```python
from build123d import *

# Parameters (mm, degrees)
SKETCH1_R           = 69.948062861
BOSS_EXTRUDE1_DEPTH = 25.4
BOSS_EXTRUDE2_DEPTH = 25.4


with BuildPart() as part:
    # Sketch1 → Boss-Extrude1 (new body)
    with BuildSketch(Plane(origin=(0, 0, 0), x_dir=(1, 0, 0), z_dir=(0, 1, 0))):
        with BuildLine():
            ThreePointArc((63.74187476, -40.530752622), (65.16096079, -41.118557302), (66.58004682, -40.530752622))
            ThreePointArc((66.58004682, -40.530752622), (14.23733744, 76.635127489), (-76.694663108, -13.913058378))
            Line((-76.694663108, -13.913058378), (-73.000086536, -13.913058378))
            Line((-73.000086536, -13.913058378), (-75.252390768, -15.474368763))
            Line((-75.252390768, -15.474368763), (-70.740426062, -15.474368763))
            Line((-70.740426062, -15.474368763), (-70.080138544, -17.015039639))
            Line((-70.080138544, -17.015039639), (-72.166015782, -17.521478191))
            Line((-72.166015782, -17.521478191), (-71.123077163, -18.775806353))
            Line((-71.123077163, -18.775806353), (-70.740426062, -20.351838073))
            Line((-70.740426062, -20.351838073), (-71.268418719, -21.218426764))
            Line((-71.268418719, -21.218426764), (-72.996408415, -24.608346096))
            Line((-72.996408415, -24.608346096), (-73.573552306, -25.740569997))
            ThreePointArc((-73.573552306, -25.740569997), (-15.15436006, -76.459073457), (58.193519931, -51.857099617))
            Line((58.193519931, -51.857099617), (58.193519931, -44.265552602))
            Line((58.193519931, -44.265552602), (60.00707478, -44.265552602))
            Line((60.00707478, -44.265552602), (63.74187476, -40.530752622))
        make_face()
        with Locations(Location((0, 0, 0), (0, 0, 90))):
            Circle(SKETCH1_R, mode=Mode.SUBTRACT)
    extrude(amount=BOSS_EXTRUDE1_DEPTH)

    # Sketch2 → Boss-Extrude2 (add)
    with BuildSketch(Plane.XZ):
        with BuildLine():
            Line((16.91938422, -42.867763876), (15.301396265, -46.734397981))
            Line((15.301396265, -46.734397981), (23.266647688, -65.965101405))
            ThreePointArc((23.266647688, -65.965101405), (27.508582432, -64.311813771), (31.633980927, -62.386078164))
            Line((31.633980927, -62.386078164), (22.646440609, -42.05853708))
            Line((22.646440609, -42.05853708), (22.122487474, -44.43690451))
            Line((22.122487474, -44.43690451), (19.98105683, -41.085378254))
            Line((19.98105683, -41.085378254), (19.154678805, -40.246982073))
            Line((19.154678805, -40.246982073), (19.154678805, -42.867763876))
            Line((19.154678805, -42.867763876), (17.562717892, -44.43690451))
            Line((17.562717892, -44.43690451), (16.91938422, -42.867763876))
        make_face()
        with BuildLine():
            Line((7.295677294, -27.358886688), (14.085059503, -43.790609078))
            Line((14.085059503, -43.790609078), (14.802816622, -40.246982073))
            Line((14.802816622, -40.246982073), (16.254758128, -40.541070969))
            Line((16.254758128, -40.541070969), (16.507439862, -39.293560089))
            Line((16.507439862, -39.293560089), (17.562717892, -39.293560089))
            Line((17.562717892, -39.293560089), (17.562717892, -38.21621684))
            Line((17.562717892, -38.21621684), (19.98105683, -38.7060483))
            Line((19.98105683, -38.7060483), (20.801456059, -37.88564907))
            Line((20.801456059, -37.88564907), (12.224600097, -18.486972039))
            ThreePointArc((12.224600097, -18.486972039), (17.735408563, -13.291511043), (21.175132345, -6.543909602))
            Line((21.175132345, -6.543909602), (68.757486976, -12.850660789))
            ThreePointArc((68.757486976, -12.850660789), (69.448887589, -8.341673136), (69.844918996, -3.797207976))
            Line((69.844918996, -3.797207976), (22.122487474, 1.343328216))
            ThreePointArc((22.122487474, 1.343328216), (20.3784905, 8.713558841), (16.254758128, 15.066247738))
            Line((16.254758128, 15.066247738), (22.122487474, 22.699365292))
            Line((22.122487474, 22.699365292), (22.122487474, 30.322912753))
            Line((22.122487474, 30.322912753), (17.562717892, 30.322912753))
            Line((17.562717892, 30.322912753), (9.897887376, 19.830300255))
            ThreePointArc((9.897887376, 19.830300255), (2.643081937, 22.005069884), (-4.920374217, 21.610157341))
            Line((-4.920374217, 21.610157341), (-16.826086698, 50.424467144))
            Line((-16.826086698, 50.424467144), (-17.435403285, 50.17270515))
            Line((-17.435403285, 50.17270515), (-19.742011126, 52.479312991))
            Line((-19.742011126, 52.479312991), (-20.850502701, 50.169534038))
            Line((-20.850502701, 50.169534038), (-23.249744789, 47.77029195))
            Line((-23.249744789, 47.77029195), (-24.874918704, 47.098790412))
            Line((-24.874918704, 47.098790412), (-12.224600097, 18.486972039))
            ThreePointArc((-12.224600097, 18.486972039), (-17.735408563, 13.291511043), (-21.175132345, 6.543909602))
            Line((-21.175132345, 6.543909602), (-68.757486976, 12.850660789))
            ThreePointArc((-68.757486976, 12.850660789), (-69.448887589, 8.341673136), (-69.844918996, 3.797207976))
            Line((-69.844918996, 3.797207976), (-22.122487474, -1.343328216))
            ThreePointArc((-22.122487474, -1.343328216), (-20.3784905, -8.713558841), (-16.254758128, -15.066247738))
            Line((-16.254758128, -15.066247738), (-45.507742187, -53.120400027))
            ThreePointArc((-45.507742187, -53.120400027), (-41.94854464, -55.973664348), (-38.210938069, -58.588870188))
            Line((-38.210938069, -58.588870188), (-9.897887376, -19.830300255))
            ThreePointArc((-9.897887376, -19.830300255), (-6.593278337, -21.159812463), (-3.118363368, -21.942761737))
            Line((-3.118363368, -21.942761737), (0, -18.824398369))
            Line((0, -18.824398369), (2.927922909, -18.824398369))
            Line((2.927922909, -18.824398369), (4.920374217, -12.850660789))
            Line((4.920374217, -12.850660789), (7.924997395, -20.697908083))
            Line((7.924997395, -20.697908083), (7.295677294, -27.358886688))
        make_face()
        with BuildLine():
            ThreePointArc((-23.249744789, 65.971060816), (-27.500342949, 64.315337484), (-31.633980927, 62.386078164))
            Line((-31.633980927, 62.386078164), (-27.537289867, 53.120400027))
            Line((-27.537289867, 53.120400027), (-21.929290512, 53.120400027))
            Line((-21.929290512, 53.120400027), (-21.929290512, 54.528885617))
            Line((-21.929290512, 54.528885617), (-21.175132345, 56.232852652))
            Line((-21.175132345, 56.232852652), (-18.874010019, 55.380869134))
            Line((-18.874010019, 55.380869134), (-23.249744789, 65.971060816))
        make_face()
        with BuildLine():
            Line((26.56555805, 28.479195616), (45.507742187, 53.120400027))
            ThreePointArc((45.507742187, 53.120400027), (41.94854464, 55.973664348), (38.210938069, 58.588870188))
            Line((38.210938069, 58.588870188), (22.122487474, 36.564915784))
            Line((22.122487474, 36.564915784), (24.054412722, 32.87896942))
            Line((24.054412722, 32.87896942), (25.891298269, 32.87896942))
            Line((25.891298269, 32.87896942), (25.891298269, 30.109133149))
            Line((25.891298269, 30.109133149), (26.56555805, 28.479195616))
        make_face()
    extrude(amount=-BOSS_EXTRUDE2_DEPTH)


solid = part.part
```
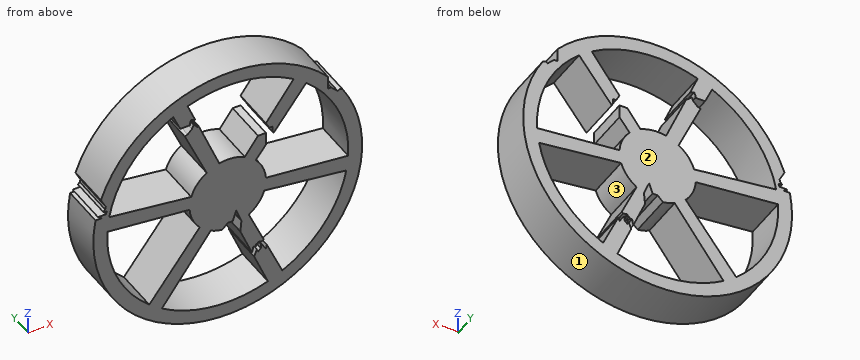
Model file for the job. Use its own axes, mm. Face numbers are marked on the shaded views. Coordinates: 2 decimals unless noted, no trailing zeros. Order: outer loops, then holes, each group sorted by start corner. A loop starts at its lowest first (then second) coordinate and runs counter-clockwise, first axis right, second up. Notation, with made-up numbers: (44, 83.25) -> (78, 83.25) arc R12 cw to (78, 105.25) -> close; hole circle Ø5 at (1, 44). An arc over 180 degrees is marked (long way). Return JSON: item names as keys, results as strings.
Item 1: Pin check, flat tips, straight feed: P1, Ø1, axis at y = 18, z = -51.5, coming from the +X side; P2, Ø8, axis at x = 6, z = -3, coming from the -Y side; P3, Ø1, axis at x = -12.5, y = 9, coming from the +Z side; P4, Ø3, axis at y = 11, z = 3.5, coming from the +X side. Stop position of each tip, or through.
Model answer:
{"P1": "stops at x = 58.95", "P2": "stops at y = 0", "P3": "stops at z = 77.02", "P4": "stops at x = 77.92"}
Item 2: Slice it at B-B (y = 10.5). Count the separate pieces of the cut face and the enclosed holes in it, then the cut area to 3 significant figures.
Model answer:
{"separate pieces": "1", "enclosed holes": "3", "area": "7,460 mm²"}
Item 3: Mould opens along Z. For the marked faces 1, 2 and 3 say: pulls with the +Z half, pulls with the -Z half, needs draft (parallel to the pull), parting line crosses it, or undercut.
Model answer:
{"face 1": "parting line crosses it", "face 2": "needs draft", "face 3": "undercut"}
Item 4: Wall check: line 1 along Z through (x, y) = (1, 14.25); line 2 along Z through (x, y) = (11, 6.5); line 3 along X through (y, z) = (19.5, -59). Give the ranges that are in metal, low to high. Write a range as from..to.
Model answer:
{"line 1": "z = -77.94..-69.94, -18.82..22.14, 69.94..77.94", "line 2": "z = -77.17..-69.08, -36.32..21.34, 69.08..77.17", "line 3": "x = -50.94..-37.57, 20.38..30.14, 37.57..50.94"}
Item 5: Slice it at A-A (x = 54.5). Write the cut outline in (y, z), then the cut area to 3 significant figures.
Model answer:
{"outline": "(0, -55.73) -> (25.4, -55.73) -> (25.4, -43.85) -> (0, -43.85) -> close; (0, -10.96) -> (25.4, -10.96) -> (25.4, -2.14) -> (0, -2.14) -> close; (0, 43.85) -> (25.4, 43.85) -> (25.4, 55.73) -> (0, 55.73) -> close", "area": "827 mm²"}
